Here's how the part is built. I have some questions about the finished solid (model axes, mm). Give positions to 0.01 mm unless a question says otherwise; leave off trailing zeros. Write each loop counter-clockwise with the first axis right and the second up, starting at its lowest first coordinate (ties: lowest second). Pieces come first, ordered by that corner, then holes. Notation, with made-up numbers: (77, 54) - (100, 54) arc R28 ccw to (100, 83) - close; hole circle Ø11 at (45.25, 69.25). An arc over 180 degrees is marked (long way). One line per item, written item: value. Start each with the question number.
1) Imagine slicing it at D-D on z = 61. Write out the boundary of the cut face in (x, y), plus the area to 3 significant figures.
2) I'm going to push flat-ended pins straight in: P1, Ø1.5, axis at x = 3, z = 33.5, coming from the -Y side; P2, Ø4, axis at x = 8, y = 15, coming from the +Z side; P3, Ø19, axis at y = -66.74, z = 48.49, coming from the +X side; P4, Ø6, axis at x = 4.5, y = -24.5, coming from the -Z side. Where does each tip first touch, or does it pass through?
3) Imagine slicing it at A-A on y = 24.5. Write out the boundary of the cut face in (x, z).
4) Imagine slicing it at B-B on y = 82.5. Write out the boundary of the cut face in (x, z).
5) Please list where these lines run through material, in increasing order: L1, parallel to Z at x = 5.75, y = 24; L2, parallel to Y at x = 5.75, z = -80; L3, parallel to Z at x = 3.5, y = 83. Write a range as [from, to].
Autodesk Inventor part; units mm, degrees
ref_plane "YZ Plane" through (0, 0, 0) normal (1, 0, 0) x (0, 1, 0)
ref_plane "XZ Plane" through (0, 0, 0) normal (0, 1, 0) x (-1, 0, 0)
ref_plane "XY Plane" through (0, 0, 0) normal (0, 0, 1) x (1, 0, 0)
sketch "Sketch1" plane through (0, 0, 0) normal (1, 0, 0) x (0, 1, 0)
  circle A0 centre (0, 0) radius 90
  dimension "d0" = 180
extrude "Extrusion1" add sketch "Sketch1" along normal blind 10
sketch "Sketch2" plane through (10, 0, 0) normal (1, 0, 0) x (0, 0, -1)
  circle A0 centre (0, 82.5) radius 6
  point P0 (0, 0)
  dimension "d3" = 82.5
  dimension "d4" = 12
extrude "Extrusion2" cut sketch "Sketch2" against normal blind 10
pattern_circular "Circular Pattern1" count 5 over 360 about axis through (10, 0, 0) along (1, 0, 0) of "Extrusion2"
properties part number "lip plate"
Numbers:
1. outline: (0, -66.17) - (10, -66.17) - (10, 66.17) - (0, 66.17) - close
1. area: 1,320 mm^2
2. P1: y = -83.83
2. P2: z = 89.06
2. P3: x = 10
2. P4: z = -87.39
3. outline: (0, -86.6) - (10, -86.6) - (10, -84.38) - (0, -84.38) - close; (0, -72.55) - (10, -72.55) - (10, 72.55) - (0, 72.55) - close; (0, 84.38) - (10, 84.38) - (10, 86.6) - (0, 86.6) - close
4. outline: (0, -35.97) - (10, -35.97) - (10, -6) - (0, -6) - close; (0, 6) - (10, 6) - (10, 35.97) - (0, 35.97) - close
5. L1: [-86.74, -84.27], [-72.65, 72.65], [84.27, 86.74]
5. L2: [-41.23, 19.69], [31.29, 41.23]
5. L3: [-34.8, -5.98], [5.98, 34.8]
